```python
from build123d import *

# Parameters (mm, degrees)
SKETCH_R   = 62.5
SKETCH_R_2 = 11
SKETCH_R_3 = 3
PAD_DEPTH  = 1.3


with BuildPart() as part:
    # Sketch → Pad (new body)
    with BuildSketch(Plane.XY):
        Circle(SKETCH_R)
        Circle(SKETCH_R_2, mode=Mode.SUBTRACT)
        with Locations((0, 46)):
            Circle(SKETCH_R_3, mode=Mode.SUBTRACT)
        with Locations((29.56823, 35.238044)):
            Circle(SKETCH_R_3, mode=Mode.SUBTRACT)
        with Locations((45.301157, 7.987816)):
            Circle(SKETCH_R_3, mode=Mode.SUBTRACT)
        with Locations((39.837169, -23)):
            Circle(SKETCH_R_3, mode=Mode.SUBTRACT)
        with Locations((15.732927, -43.225861)):
            Circle(SKETCH_R_3, mode=Mode.SUBTRACT)
        with Locations((-15.732927, -43.225861)):
            Circle(SKETCH_R_3, mode=Mode.SUBTRACT)
        with Locations((-39.837169, -23)):
            Circle(SKETCH_R_3, mode=Mode.SUBTRACT)
        with Locations((-45.301157, 7.987816)):
            Circle(SKETCH_R_3, mode=Mode.SUBTRACT)
        with Locations((-29.56823, 35.238044)):
            Circle(SKETCH_R_3, mode=Mode.SUBTRACT)
    extrude(amount=PAD_DEPTH)


solid = part.part
```
Design review of the part built by this model. Coordinates are the model's own, in mm. Give positions to 0.01 mm unless a question says otherwise; leave off trailing zeros. Write each loop counter-clockwise with the first axis right and the second up, starting at its lowest first coordinate (ties: lowest second). Pieces come first, ordered by that corner, then holes. Notation, with made-up numbers: (29, -7) -> (41, -7) arc R11 ccw to (41, 1) -> close; hole circle Ø2 at (70, -37.75). An arc over 180 degrees is marked (long way). Answer in a Markdown table with one row per item.
(1) To check wall thickness, follow probe 1 along Y at (x, z) = (0, 1); probe 2 along X at (y, z) = (7, 0.45); probe 3 along X at (y, z) = (36.5, 0.65). State the ranges of each line that lie inside material, in increasing order.
Results:
| item | result |
|---|---|
| probe 1 | -62.5 to -11, 11 to 43, 49 to 62.5 |
| probe 2 | -62.11 to -48.13, -42.47 to -8.49, 8.49 to 42.47, 48.13 to 62.11 |
| probe 3 | -50.73 to -32.29, -26.85 to 26.85, 32.29 to 50.73 |
(2) Consider section C-C (z = 1.1). Count the separate pieces of the cut face and the enclosed holes in it, then the cut area to 3 significant figures.
Results:
| item | result |
|---|---|
| separate pieces | 1 |
| enclosed holes | 10 |
| area | 11,600 mm2 |
(3) Mouldability with a two-part tool opening along Y and no side actions: class faces 1 (the flat face through (13, 1, 0)), 2 (the cylindrical face through (-26.707, 36.139, 0.641)), 3 (the cylindrical face through (-62.44, 2.75, 0.64)) as +Y half, -Y half, draft (parallel to the pull), parting line (faces both ways), or undercut.
Results:
| item | result |
|---|---|
| face 1 | draft |
| face 2 | undercut |
| face 3 | parting line |
(4) Consider section A-A (y = 0). State the section outline as (x, z) points, then the cut area to 3 significant figures.
Results:
| item | result |
|---|---|
| outline | (-62.5, 0) -> (-11, 0) -> (-11, 1.3) -> (-62.5, 1.3) -> close; (11, 0) -> (62.5, 0) -> (62.5, 1.3) -> (11, 1.3) -> close |
| area | 134 mm2 |
(5) Consider section D-D (y = -23). State the section outline as (x, z) points.
Results:
| item | result |
|---|---|
| outline | (-58.11, 0) -> (-42.84, 0) -> (-42.84, 1.3) -> (-58.11, 1.3) -> close; (-36.84, 0) -> (36.84, 0) -> (36.84, 1.3) -> (-36.84, 1.3) -> close; (42.84, 0) -> (58.11, 0) -> (58.11, 1.3) -> (42.84, 1.3) -> close |
(6) Consider section B-B (x = 0). State the section outline as (y, z) points, then the cut area to 3 significant figures.
Results:
| item | result |
|---|---|
| outline | (-62.5, 0) -> (-11, 0) -> (-11, 1.3) -> (-62.5, 1.3) -> close; (11, 0) -> (43, 0) -> (43, 1.3) -> (11, 1.3) -> close; (49, 0) -> (62.5, 0) -> (62.5, 1.3) -> (49, 1.3) -> close |
| area | 126 mm2 |
